The listing builds one solid part. Answer for the finished solid, in the listing's coordinates (mm). A direction names the side the tool comes from. Give positions to 0.01 mm unless a question says otherwise; leave off trailing zeros. Order: outer loops, then holes, each group sorted by start corner. A loop starts at its lowest first (then second) coordinate and runs counter-clockwise, first axis right, second up. Notation, with made-up numbers: (69.5, -5) -> (109.5, -5) arc R13 cw to (109.5, 18) -> close; hole circle Ø9 at (79.25, 34.25). An arc over 180 degrees is marked (long way). Answer as a JSON object with one key per item and string values. Group by question number.
```python
from build123d import *

# Parameters (mm, degrees)
SKETCH_W     = 50
SKETCH_H     = 43
SKETCH_R     = 15
SKETCH_R_2   = 2
PAD_DEPTH    = 5
SKETCH001_W  = 9
SKETCH001_H  = 2
PAD001_DEPTH = 17
SKETCH002_R  = 2
POCKET_DEPTH = 11


with BuildPart() as part:
    # Sketch → Pad (new body)
    with BuildSketch(Plane.XY):
        with Locations((25, 21.5)):
            Rectangle(SKETCH_W, SKETCH_H)
        with Locations((24, 22.2)):
            Circle(SKETCH_R, mode=Mode.SUBTRACT)
        with Locations((40, 38.2)):
            Circle(SKETCH_R_2, mode=Mode.SUBTRACT)
        with Locations((8, 38.2)):
            Circle(SKETCH_R_2, mode=Mode.SUBTRACT)
        with Locations((8, 6.2)):
            Circle(SKETCH_R_2, mode=Mode.SUBTRACT)
        with Locations((40, 6.2)):
            Circle(SKETCH_R_2, mode=Mode.SUBTRACT)
    extrude(amount=PAD_DEPTH)

    # Sketch001 → Pad001 (join)
    with BuildSketch(Plane.XY):
        with Locations((45.5, 10.5)):
            Rectangle(SKETCH001_W, SKETCH001_H)
        with Locations((4.5, 10.5)):
            Rectangle(SKETCH001_W, SKETCH001_H)
        with Locations((4.5, 18.5)):
            Rectangle(SKETCH001_W, SKETCH001_H)
        with Locations((45.5, 18.5)):
            Rectangle(SKETCH001_W, SKETCH001_H)
    extrude(amount=-PAD001_DEPTH)

    # Sketch002 (on Face10 of Pad001) → Pocket (cut)
    with BuildSketch(Plane(origin=(0, 19.5, 0), x_dir=(-1, 0, 0), z_dir=(0, 1, 0))):
        with Locations((-5, -6)):
            Circle(SKETCH002_R)
        with Locations((-45, -6)):
            Circle(SKETCH002_R)
    extrude(amount=-POCKET_DEPTH, mode=Mode.SUBTRACT)


solid = part.part
```
(1) Which of the six approach directions +Z, -Z, +X, -X, +Y, -Y give full straight-line access (tool end or side, diameter ignored) to faces 4 (the flat face through (41, 18, -8)), 5 (the flat face through (45.4, 19.5, -8.4)), 6 (the flat face through (25, 43, 2)), 7 (the flat face through (45.4, 11.5, -8.4))?
(2) Find the intervals of material crossed by line 1 along Y through (x, z) = (47, -2.5); line 2 along Y through (x, z) = (40, 1.3); line 3 along Z through (x, y) = (45, 10), in increasing order. Write a range as [from, to].
(3) Flat-ended cylindrical pins translate along their axes: pin 1 Ø7 at (x, z) = (6.5, -10) entering from +Y; pin 2 Ø5 at (x, y) = (7.5, 35.5) entering from -Z; pin 3 Ø10 at (x, z) = (44.5, -8) entering from -Y. Find the tip coordinate at first contact, or state that the pin passes through.
(4) A cutting plane is placed at C-C (z = -10.75). Determine the outline of the cut face in (x, y).
(5) For a pull along Z with two mould halves and no side action, classify faces 1 (the flat face through (4, 19.5, -8)), 2 (the flat face through (45, 11, -17)), 3 (the cylindrical face through (47, 19, -6)) as +Z half, -Z half, draft (parallel to the pull), parting line (faces both ways), or undercut.
(6) A cutting plane is placed at D-D (y = 38.2). Determine the outline of the cut face in (x, z), and give its area (3 significant figures).
(7) A cutting plane is placed at B-B (x = 45). Determine the outline of the cut face in (y, z).
(8) A cutting plane is placed at A-A (y = 22.2). Determine the outline of the cut face in (x, z).
Check sheet entries:
{
 "1": {"face 4": "-Z, +Y, -Y", "face 5": "-Z, +X, -X, +Y", "face 6": "+Z, -Z, +X, -X, +Y", "face 7": "-Z, +X, -X"},
 "2": {"line 1": "y = [9.5, 11.5], [17.5, 19.5]", "line 2": "y = [0, 4.2], [8.2, 36.2], [40.2, 43]", "line 3": "z = [-17, -8], [-4, 5]"},
 "3": {"pin 1": "stops at y = 19.5", "pin 2": "stops at z = 0", "pin 3": "stops at y = 9.5"},
 "4": {"outline": "(0, 9.5) -> (9, 9.5) -> (9, 11.5) -> (0, 11.5) -> close; (0, 17.5) -> (9, 17.5) -> (9, 19.5) -> (0, 19.5) -> close; (41, 9.5) -> (50, 9.5) -> (50, 11.5) -> (41, 11.5) -> close; (41, 17.5) -> (50, 17.5) -> (50, 19.5) -> (41, 19.5) -> close"},
 "5": {"face 1": "draft", "face 2": "-Z half", "face 3": "undercut"},
 "6": {"outline": "(0, 0) -> (6, 0) -> (6, 5) -> (0, 5) -> close; (10, 0) -> (38, 0) -> (38, 5) -> (10, 5) -> close; (42, 0) -> (50, 0) -> (50, 5) -> (42, 5) -> close", "area": "210 mm2"},
 "7": {"outline": "(0, 0) -> (9.5, 0) -> (9.5, -4) -> (11.5, -4) -> (11.5, 0) -> (17.5, 0) -> (17.5, -4) -> (19.5, -4) -> (19.5, 0) -> (43, 0) -> (43, 5) -> (0, 5) -> close; (9.5, -17) -> (11.5, -17) -> (11.5, -8) -> (9.5, -8) -> close; (17.5, -17) -> (19.5, -17) -> (19.5, -8) -> (17.5, -8) -> close"},
 "8": {"outline": "(0, 0) -> (9, 0) -> (9, 5) -> (0, 5) -> close; (39, 0) -> (50, 0) -> (50, 5) -> (39, 5) -> close"}
}
